```python
from build123d import *

# Parameters (mm, degrees)
BOSS_EXTRUDE2_DEPTH     = 5
CHAMFER2_SIZE           = 2
CUT_EXTRUDE2_DEPTH      = 4
CUT_EXTRUDE2_DEPTH_BACK = 14
SKETCH3_W               = 9
SKETCH3_H               = 5
SKETCH3_W_2             = 6.574069069
SKETCH3_W_3             = 2.425930931
SKETCH4_R               = 2.1
CUT_EXTRUDE3_DEPTH      = 85.075405536
CHAMFER3_SIZE           = 2


with BuildPart() as part:
    # Sketch1 → Boss-Extrude2 (new, symmetric)
    with BuildSketch(Plane.XY):
        with BuildLine():
            Line((-70.627945664, 2.425930931), (-75, 0))
            Line((-75, 0), (-70, 0))
            ThreePointArc((-70, 0), (-70.159531444, 1.252942201), (-70.627945664, 2.425930931))
        make_face()
        with BuildLine():
            Line((-70, 0), (-75, 0))
            Line((-75, 0), (-70.627945664, 2.425930931))
            ThreePointArc((-70.627945664, 2.425930931), (-72.463235787, 4.308692067), (-75, 5))
            ThreePointArc((-75, 5), (-79.372054336, -2.425930931), (-70.757479261, -2.645943647))
            ThreePointArc((-70.757479261, -2.645943647), (-70.193098519, -1.376117057), (-70, 0))
        make_face()
        with BuildLine():
            ThreePointArc((-75, 5), (-72.463235787, 4.308692067), (-70.627945664, 2.425930931))
            Line((-70.627945664, 2.425930931), (-46.692296896, 15.707154411))
            ThreePointArc((-46.692296896, 15.707154411), (-38.703947646, 18.501488579), (-30.241024495, 18.470522187))
            Line((-30.241024495, 18.470522187), (70.075272109, 0.864323549))
            ThreePointArc((70.075272109, 0.864323549), (71.784538738, 3.828943571), (75, 5))
            Line((75, 5), (-30.241024495, 23.470522187))
            ThreePointArc((-30.241024495, 23.470522187), (-38.703947646, 23.501488579), (-46.692296896, 20.707154411))
            Line((-46.692296896, 20.707154411), (-75, 5))
        make_face()
        with BuildLine():
            ThreePointArc((-70.627945664, 2.425930931), (-70.159531444, 1.252942201), (-70, 0))
            Line((-70, 0), (-65.988914235, 0))
            Line((-65.988914235, 0), (-46.692296896, 10.707154411))
            ThreePointArc((-46.692296896, 10.707154411), (-38.703947646, 13.501488579), (-30.241024495, 13.470522187))
            Line((-30.241024495, 13.470522187), (46.511085765, 0))
            Line((46.511085765, 0), (70, 0))
            ThreePointArc((70, 0), (70.018853573, 0.433797501), (70.075272109, 0.864323549))
            Line((70.075272109, 0.864323549), (-30.241024495, 18.470522187))
            ThreePointArc((-30.241024495, 18.470522187), (-38.703947646, 18.501488579), (-46.692296896, 15.707154411))
            Line((-46.692296896, 15.707154411), (-70.627945664, 2.425930931))
        make_face()
        with BuildLine():
            ThreePointArc((70.075272109, 0.864323549), (70.018853573, 0.433797501), (70, 0))
            Line((70, 0), (75, 0))
            Line((75, 0), (70.075272109, 0.864323549))
        make_face()
        with BuildLine():
            Line((75, 0), (70, 0))
            ThreePointArc((70, 0), (70.90652247, -2.871139445), (73.297376685, -4.701177921))
            ThreePointArc((73.297376685, -4.701177921), (77.871139445, -4.09347753), (80, 0))
            ThreePointArc((80, 0), (78.535533906, 3.535533906), (75, 5))
            ThreePointArc((75, 5), (71.784538738, 3.828943571), (70.075272109, 0.864323549))
            Line((70.075272109, 0.864323549), (75, 0))
        make_face()
        with BuildLine():
            Line((70, 0), (46.511085765, 0))
            Line((46.511085765, 0), (73.297376685, -4.701177921))
            ThreePointArc((73.297376685, -4.701177921), (70.90652247, -2.871139445), (70, 0))
        make_face()
        with BuildLine():
            Line((-65.988914235, 0), (-70, 0))
            ThreePointArc((-70, 0), (-70.193098519, -1.376117057), (-70.757479261, -2.645943647))
            Line((-70.757479261, -2.645943647), (-65.988914235, 0))
        make_face()
        with BuildLine():
            Line((-70.627945664, 2.425930931), (-75, 0))
            Line((-75, 0), (-70, 0))
            ThreePointArc((-70, 0), (-70.159531444, 1.252942201), (-70.627945664, 2.425930931))
        make_face()
        with BuildLine():
            Line((-70, 0), (-75, 0))
            Line((-75, 0), (-70.627945664, 2.425930931))
            ThreePointArc((-70.627945664, 2.425930931), (-72.463235787, 4.308692067), (-75, 5))
            ThreePointArc((-75, 5), (-79.372054336, -2.425930931), (-70.757479261, -2.645943647))
            ThreePointArc((-70.757479261, -2.645943647), (-70.193098519, -1.376117057), (-70, 0))
        make_face()
        with BuildLine():
            ThreePointArc((70.075272109, 0.864323549), (70.018853573, 0.433797501), (70, 0))
            Line((70, 0), (75, 0))
            Line((75, 0), (70.075272109, 0.864323549))
        make_face()
        with BuildLine():
            Line((75, 0), (70, 0))
            ThreePointArc((70, 0), (70.90652247, -2.871139445), (73.297376685, -4.701177921))
            ThreePointArc((73.297376685, -4.701177921), (77.871139445, -4.09347753), (80, 0))
            ThreePointArc((80, 0), (78.535533906, 3.535533906), (75, 5))
            ThreePointArc((75, 5), (71.784538738, 3.828943571), (70.075272109, 0.864323549))
            Line((70.075272109, 0.864323549), (75, 0))
        make_face()
    extrude(amount=BOSS_EXTRUDE2_DEPTH, both=True)

    # Chamfer2
    chamfer2_edges = [part.edges().sort_by_distance(p)[0] for p in [
        (-38.703947646, 13.501488579, -5),
        (-58.724888079, 4.030605382, -5),
        (-79.372054336, -2.425930931, -5),
        (-60.846148448, 12.853577206, -5),
        (-38.703947646, 23.501488579, -5),
        (22.379487752, 14.235261094, -5),
        (79.924727891, -0.864323549, -5),
        (21.528176095, 4.384672133, -5),
    ]]
    chamfer(chamfer2_edges, length=CHAMFER2_SIZE)

    # Sketch3 → Cut-Extrude2 (cut, two sides: drawn at the far end of the back side and taken through both)
    with BuildSketch(Plane(origin=(-19.776683018, 35.641877363, 0), x_dir=(0.8744108672058327, 0.48518618623405146, 0), z_dir=(-0.48518618623405146, 0.8744108672058327, 0)).offset(-CUT_EXTRUDE2_DEPTH_BACK)):
        with Locations((-70.08081504, 0)):
            Rectangle(SKETCH3_W, SKETCH3_H)
        with Locations((-59.867849574, 0)):
            Rectangle(SKETCH3_W_2, SKETCH3_H)
        with Locations((-64.367849574, 0)):
            Rectangle(SKETCH3_W_3, SKETCH3_H)
    extrude(amount=CUT_EXTRUDE2_DEPTH + CUT_EXTRUDE2_DEPTH_BACK, mode=Mode.SUBTRACT)

    # Sketch4 → Cut-Extrude3 (cut, through all)
    with BuildSketch(Plane.XY.offset(5)):
        with Locations((-75, 0)):
            Circle(SKETCH4_R)
        with Locations((75, 0)):
            Circle(SKETCH4_R)
    extrude(amount=-CUT_EXTRUDE3_DEPTH, mode=Mode.SUBTRACT)

    # Chamfer3
    chamfer3_edges = [part.edges().sort_by_distance(p)[0] for p in [
        (79.924727891, -0.864323549, 5),
        (22.379487752, 14.235261094, 5),
        (-38.703947646, 23.501488579, 5),
        (-60.846148448, 12.853577206, 5),
        (-79.372054336, -2.425930931, 5),
        (21.528176095, 4.384672133, 5),
        (-58.724888079, 4.030605382, 5),
        (-38.703947646, 13.501488579, 5),
    ]]
    chamfer(chamfer3_edges, length=CHAMFER3_SIZE)


solid = part.part
```
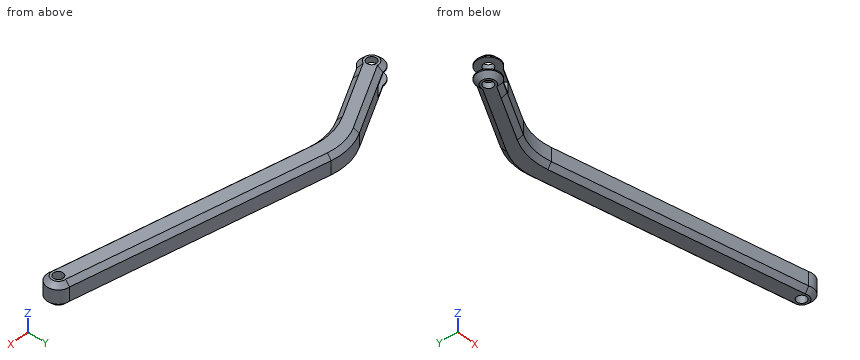
Model file for the job. Use its own axes, mm. Coordinates: 2 decimals unless noted, no trailing zeros. Order: outer loops, then holes, each group sorted by start corner. A loop starts at its lowest first (then second) coordinate and runs counter-clockwise, first axis right, second up. Notation, with made-up numbers: (-33.5, 36) -> (-6.5, 36) arc R10 cw to (-6.5, 47) -> close; hole circle Ø4 at (49, -37.75). An arc over 180 degrees is marked (long way). Return JSON: item names as keys, results as strings.
Item 1: Wall check: line 1 along Y through (x, z) = (-75, 3.65); line 2 along Y through (x, z) = (-75, -3.35); line 3 along Y through (x, z) = (5, -4). Give the ranges that are in metal, low to high. Write a range as from..to.
Model answer:
{"line 1": "y = -4.35..-2.1, 2.1..4.35", "line 2": "y = -4.65..-2.1, 2.1..4.65", "line 3": "y = 8.3..16.27"}
Item 2: Slice it at B-B (x = 62). Write the cut outline in (y, z).
Model answer:
{"outline": "(-2.72, -3) -> (-0.69, -5) -> (5.25, -5) -> (7.28, -3) -> (7.28, 3) -> (5.25, 5) -> (-0.69, 5) -> (-2.72, 3) -> close"}
Item 3: Pin check, flat tips, straight feed: P1, Ø4, axis at x = 75, y = 0, coming from the +Z side; P2, Ø1.5, axis at y = 17.5, z = 3, coming from the -X side; P3, Ø3, axis at y = 9, z = -3, coming from the -X side; P4, Ø6, axis at y = 15, z = -0.5, coming from the -X side. Stop position of each tip, or through.
Model answer:
{"P1": "passes through", "P2": "stops at x = -53.82", "P3": "stops at x = -70.49", "P4": "stops at x = -62.38"}
Item 4: Slice it at A-A (z = 1). Write the cut outline in (x, y), then the cut area to 3 significant figures.
Model answer:
{"outline": "(-69.25, 8.19) -> (-65.01, 0.54) -> (-46.69, 10.71) arc R25 cw to (-30.24, 13.47) -> (73.3, -4.7) arc R5 ccw (long way) to (75, 5) -> (-30.24, 23.47) arc R25 ccw to (-46.69, 20.71) -> close; hole circle Ø4.2 at (75, 0)", "area": "1,450 mm²"}
